Study the drawing (mm; zero at the part's minimum x, y, z) and answer. A direction names the side the tool comes from. Give positions to 0.01 mm unless a question says otherwise; leave off trailing zeros. Loops run counter-clockwise (first coordinate to the right, second up) from the corner with the lowest first, then second, coordinate; pieces in that order, holes last. Notation, with made-up numbers: M 9.5,81.25 L 30.5,81.25 A25 cw 30.5,115.25 Z; hole C -11,45.25 d2. An arc over 180 degrees is marked long. Return JSON: item names as keys, results as strings.
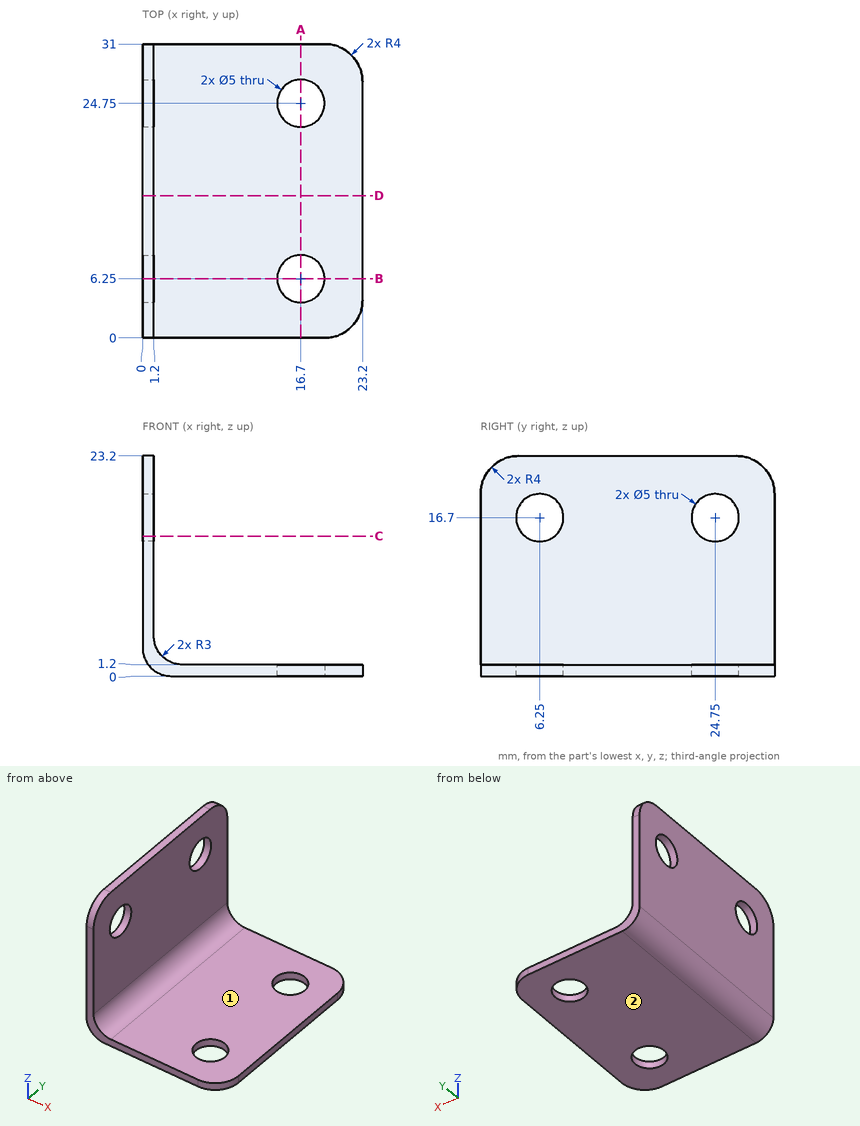
(1) The part is cut by section D-D (y = 15). Determine the outline of the cut face in (x, z).
Values follow:
{"outline": "M 0,3 A3 ccw 3,0 L 23.2,0 L 23.2,1.2 L 4.2,1.2 A3 cw 1.2,4.2 L 1.2,23.2 L 0,23.2 Z"}
(2) Straight lines are drawn through the part: line 1 along Y through (x, z) = (0.8, 16.7); line 2 along Z through (x, y) = (18.75, 12). For each, find the intervals that lie inside material, in ascending order.
Values follow:
{"line 1": "0 to 3.75, 8.75 to 22.25, 27.25 to 31", "line 2": "0 to 1.2"}
(3) The part is cut by section B-B (y = 6.25). Determine the outline of the cut face in (x, z).
Values follow:
{"outline": "M 0,3 A3 ccw 3,0 L 14.2,0 L 14.2,1.2 L 4.2,1.2 A3 cw 1.2,4.2 L 1.2,14.2 L 0,14.2 Z; M 0,19.2 L 1.2,19.2 L 1.2,23.2 L 0,23.2 Z; M 19.2,0 L 23.2,0 L 23.2,1.2 L 19.2,1.2 Z"}
(4) The part is cut by section A-A (x = 16.7). Determine the outline of the cut face in (y, z), and give its area (3 significant figures).
Values follow:
{"outline": "M 0,0 L 3.75,0 L 3.75,1.2 L 0,1.2 Z; M 8.75,0 L 22.25,0 L 22.25,1.2 L 8.75,1.2 Z; M 27.25,0 L 31,0 L 31,1.2 L 27.25,1.2 Z", "area": "25.2 mm²"}
(5) Given pin 1 (2 mm diameter, centred on x = 20.5, y = 6, fed in from +Z); pin 2 (8 mm diameter, centred on x = 5.5, y = 9.5, fed in from +Z); pin 3 (6 mm diameter, centred on y = 6.25, z = 16.7, fed in from +X); pin 4 (3 mm diameter, centred on y = 24.75, z = 16.7, fed in from +X), each flat-ended and moving along its own axis, determine where each tip first touches the part or whether it passes through.
Values follow:
{"pin 1": "z = 1.2", "pin 2": "z = 2.89", "pin 3": "x = 1.2", "pin 4": "through"}
(6) A tool of negligible diameter and unlimited length cuts with its end or side. For the marked faces 1 and 2, from which of +Z, -Z, +X, -X, +Y, -Y can it reach the whole face along a straight path? Write none if from no direction.
Values follow:
{"face 1": "+Z, +X, +Y, -Y", "face 2": "-Z, +X, -X, +Y, -Y"}
(7) The part is cut by section C-C (z = 14.75). Determine the outline of the cut face in (x, y).
Values follow:
{"outline": "M 0,0 L 1.2,0 L 1.2,4.69 L 0,4.69 Z; M 0,7.81 L 1.2,7.81 L 1.2,23.19 L 0,23.19 Z; M 0,26.31 L 1.2,26.31 L 1.2,31 L 0,31 Z"}
